from build123d import *

# Parameters (mm, degrees)
ESQUISSE1_W             = 257
ESQUISSE1_H             = 309
BOSS_EXTRU_1_DEPTH      = 3
ESQUISSE2_W             = 201
ESQUISSE2_H             = 115
ENL_V_MAT_EXTRU_1_DEPTH = 4
ENL_V_MAT_EXTRU_2_DEPTH = 4


with BuildPart() as part:
    # Esquisse1 → Boss.-Extru.1 (new body)
    with BuildSketch(Plane.XY):
        Rectangle(ESQUISSE1_W, ESQUISSE1_H)
        with BuildLine():
            Line((-114.5, 123.25), (-107.5, 123.25))
            ThreePointArc((-107.5, 123.25), (-105.75, 121.5), (-107.5, 119.75))
            Line((-107.5, 119.75), (-114.5, 119.75))
            ThreePointArc((-114.5, 119.75), (-116.25, 121.5), (-114.5, 123.25))
        make_face(mode=Mode.SUBTRACT)
        with BuildLine():
            Line((107.5, -119.75), (114.5, -119.75))
            ThreePointArc((114.5, -119.75), (116.25, -121.5), (114.5, -123.25))
            Line((114.5, -123.25), (107.5, -123.25))
            ThreePointArc((107.5, -123.25), (105.75, -121.5), (107.5, -119.75))
        make_face(mode=Mode.SUBTRACT)
        with BuildLine():
            Line((-114.5, -119.75), (-107.5, -119.75))
            ThreePointArc((-107.5, -119.75), (-105.75, -121.5), (-107.5, -123.25))
            Line((-107.5, -123.25), (-114.5, -123.25))
            ThreePointArc((-114.5, -123.25), (-116.25, -121.5), (-114.5, -119.75))
        make_face(mode=Mode.SUBTRACT)
        with BuildLine():
            Line((107.5, 123.25), (114.5, 123.25))
            ThreePointArc((114.5, 123.25), (116.25, 121.5), (114.5, 119.75))
            Line((114.5, 119.75), (107.5, 119.75))
            ThreePointArc((107.5, 119.75), (105.75, 121.5), (107.5, 123.25))
        make_face(mode=Mode.SUBTRACT)
    extrude(amount=BOSS_EXTRU_1_DEPTH)

    # Esquisse2 → Enlèv. mat.-Extru.1 (cut, through all)
    with BuildSketch(Plane.XY.offset(3)):
        with Locations((0, -97)):
            Rectangle(ESQUISSE2_W, ESQUISSE2_H)
    extrude(amount=-ENL_V_MAT_EXTRU_1_DEPTH, mode=Mode.SUBTRACT)

    # Esquisse3 → Enlèv. mat.-Extru.2 (cut, through all)
    with BuildSketch(Plane.XY.offset(3)):
        with BuildLine():
            Line((-111, 60.5), (-51, 60.5))
            ThreePointArc((-51, 60.5), (-47.464466094, 61.964466094), (-46, 65.5))
            Line((-46, 65.5), (-46, 90.5))
            ThreePointArc((-46, 90.5), (-47.464466094, 94.035533906), (-51, 95.5))
            Line((-51, 95.5), (-111, 95.5))
            ThreePointArc((-111, 95.5), (-114.535533906, 94.035533906), (-116, 90.5))
            Line((-116, 90.5), (-116, 65.5))
            ThreePointArc((-116, 65.5), (-114.535533906, 61.964466094), (-111, 60.5))
        make_face()
    extrude(amount=-ENL_V_MAT_EXTRU_2_DEPTH, mode=Mode.SUBTRACT)


solid = part.part
Geometry: final body of the model. Coordinates: model frame, mm. Coordinates: 2 decimals unless noted, no trailing zeros. Loops run counter-clockwise (first coordinate to the right, second up) from the corner with the lowest first, then second, coordinate; pieces in that order, holes last. Notation, with made-up numbers: M 31,14 L 54,14 A8 ccw 54,24 Z; hole C 1,82.25 d8. An arc over 180 degrees is marked long. One line per item, written item: value. Start each with the question number.
1) Pin query (flat end, axial travel): P1, Ø0.9, axis at x = -3, z = 2, coming from the -Y side. Return the tip coordinate at first contact, or that it passes through.
2) Material intervals for L1, parallel to Y at x = -51, z = 2; L2, parallel to X at y = -99.5, z = 0.35; L3, parallel to Y at x = -101, z = 2.5, sorted ascending. Write a range as from..to.
3) Cut plane C-C (x = -18.5). Return loops of the section in (y, z), then the cut area to 3 significant figures.
4) Cut plane A-A (z = 2.4). Count the separate pieces of the cut face and the enclosed holes in it, then the cut area to 3 significant figures.
5) Cut plane B-B (x = -69). Return loops of the section in (y, z).
Evaluation:
1. P1: y = -39.5
2. L1: -39.5..60.5, 95.5..154.5
2. L2: -128.5..-100.5, 100.5..128.5
2. L3: -154.5..60.5, 95.5..154.5
3. outline: M -39.5,0 L 154.5,0 L 154.5,3 L -39.5,3 Z
3. area: 582 mm^2
4. separate pieces: 1
4. enclosed holes: 5
4. area: 53,700 mm^2
5. outline: M -39.5,0 L 60.5,0 L 60.5,3 L -39.5,3 Z; M 95.5,0 L 154.5,0 L 154.5,3 L 95.5,3 Z
